Geometry: final body of the model. Coordinates: model frame, mm. A direction names the side the tool comes from. Coordinates: 2 decimals unless noted, no trailing zeros. Write each loop counter-clockwise with the first axis right and the second up, starting at its lowest first coordinate (ties: lowest second). Pieces come first, ordered by that corner, then holes. Notation, with made-up numbers: (13, -31) -> (64, -31) arc R16 cw to (64, 0) -> close; hole circle Ø11 at (-24.5, 67.5). An arc over 180 degrees is marked (long way). One line per item, written item: value.
```python
from build123d import *

# Parameters (mm, degrees)
SKETCH1_R           = 12.4
BOSS_EXTRUDE1_DEPTH = 7
SKETCH2_R           = 1
CUT_EXTRUDE1_DEPTH  = 19.881737208
WRAP1_START         = -0.5
WRAP1_DEPTH         = 0.5
SKETCH4_R           = 0.5
CUT_EXTRUDE2_DEPTH  = 7


# Read off the part's stored shape, not the designer's step: Wrap1
with BuildPart() as part:
    # Sketch1 → Boss-Extrude1 (new body)
    with BuildSketch(Plane(origin=(0, 0, 0), x_dir=(1, 0, 0), z_dir=(0, 1, 0))):
        with Locations(Location((0, 0, 0), (0, 0, 270))):
            Circle(SKETCH1_R)
    extrude(amount=BOSS_EXTRUDE1_DEPTH)

    # Sketch2 → Cut-Extrude1 (cut, through all)
    with BuildSketch(Plane(origin=(0, 0, 0), x_dir=(-1, 0, 0), z_dir=(0, -1, 0))):
        with Locations(Location((0, 9.7, 0), (0, 0, 90))):
            Circle(SKETCH2_R)
        with Locations(Location((0, -9.7, 0), (0, 0, 90))):
            Circle(SKETCH2_R)
    extrude(amount=-CUT_EXTRUDE1_DEPTH, mode=Mode.SUBTRACT)

    # Wrap1 outline → Wrap1 (cut)
    # profile 1 of 6: a face of its own
    with BuildSketch(Plane.XZ.offset(WRAP1_START)):
        with BuildLine():
            Line((-2.031477868, -3.153846154), (-2.210263925, -3.153846154))
            add(Edge.make_bspline(
                [(-2.210263925, -3.153846154), (-2.304050451, -3.153758336), (-2.51704944, -3.153558894), (-2.728459302, -3.180072549), (-2.846782355, -3.194911859)],
                knots=[0, 0, 0, 0, 0.440314414, 1, 1, 1, 1], degree=3))
            add(Edge.make_bspline(
                [(-2.846782355, -3.194911859), (-2.973262529, -3.243260598), (-3.258825144, -3.352420729), (-3.314541645, -3.658766612), (-3.345580432, -3.829427083)],
                knots=[0, 0, 0, 0, 0.442915733, 1, 1, 1, 1], degree=3))
            add(Edge.make_bspline(
                [(-3.345580432, -3.829427083), (-3.329443977, -3.960601874), (-3.292993392, -4.25691217), (-3.019329137, -4.388888631), (-2.866814406, -4.462439904)],
                knots=[0, 0, 0, 0, 0.442694001, 1, 1, 1, 1], degree=3))
            add(Edge.make_bspline(
                [(-2.866814406, -4.462439904), (-2.783809352, -4.4741997), (-2.595026902, -4.500945579), (-2.404280932, -4.500339561), (-2.297403348, -4.5)],
                knots=[0, 0, 0, 0, 0.439686282, 1, 1, 1, 1], degree=3))
            Line((-2.297403348, -4.5), (-1.807118893, -4.5))
            Line((-1.807118893, -4.5), (-1.807118893, -2))
            Line((-1.807118893, -2), (-2.031477868, -2))
            Line((-2.031477868, -2), (-2.031477868, -3.153846154))
        make_face()
        with BuildLine():
            Line((-2.031477868, -4.243589744), (-2.488709438, -4.243589744))
            add(Edge.make_bspline(
                [(-2.488709438, -4.243589744), (-2.636778663, -4.245832648), (-2.858668728, -4.249193765), (-3.087398478, -4.043591474), (-3.109947004, -3.900148285), (-3.121221457, -3.828425481)],
                knots=[0, 0, 0, 0, 0.500718692, 0.750355136, 1, 1, 1, 1], degree=3))
            add(Edge.make_bspline(
                [(-3.121221457, -3.828425481), (-3.110084042, -3.754426269), (-3.087818883, -3.606492103), (-2.846982746, -3.401705038), (-2.620432253, -3.403529508), (-2.469178188, -3.404747596)],
                knots=[0, 0, 0, 0, 0.249615048, 0.499013341, 1, 1, 1, 1], degree=3))
            Line((-2.469178188, -3.404747596), (-2.031477868, -3.41025641))
            Line((-2.031477868, -3.41025641), (-2.031477868, -4.243589744))
        make_face(mode=Mode.SUBTRACT)
    # profile 2 of 6: a face of its own
    with BuildSketch(Plane.XZ.offset(WRAP1_START)):
        with BuildLine():
            add(Edge.make_bspline(
                [(-1.29429838, -3.251001603), (-1.233767931, -3.555711086), (-1.13419239, -4.056973037), (-0.546785242, -4.501043755), (-0.158404316, -4.54307981), (0.035829825, -4.564102564)],
                knots=[0, 0, 0, 0, 0.436607301, 0.718240291, 1, 1, 1, 1], degree=3))
            add(Edge.make_bspline(
                [(0.035829825, -4.564102564), (0.337186775, -4.501451173), (0.832784511, -4.398417587), (1.263646175, -3.813137767), (1.310482432, -3.430401214), (1.333906748, -3.238982372)],
                knots=[0, 0, 0, 0, 0.436786424, 0.718318801, 1, 1, 1, 1], degree=3))
            add(Edge.make_bspline(
                [(1.333906748, -3.238982372), (1.271523902, -2.938761966), (1.168876948, -2.444768626), (0.592223534, -2.001267596), (0.207932181, -1.957686637), (0.015797773, -1.935897436)],
                knots=[0, 0, 0, 0, 0.436529586, 0.718281316, 1, 1, 1, 1], degree=3))
            add(Edge.make_bspline(
                [(0.015797773, -1.935897436), (-0.285288336, -1.99709136), (-0.780661114, -2.09777287), (-1.227049335, -2.673889596), (-1.271884529, -3.058652359), (-1.29429838, -3.251001603)],
                knots=[0, 0, 0, 0, 0.436613243, 0.71835368, 1, 1, 1, 1], degree=3))
        make_face()
        with BuildLine():
            add(Edge.make_bspline(
                [(0.024812197, -4.307692308), (-0.222096477, -4.260150518), (-0.627501361, -4.182090587), (-1.011681906, -3.724534497), (-1.050518548, -3.409193504), (-1.069939406, -3.251502404)],
                knots=[0, 0, 0, 0, 0.437825955, 0.718876246, 1, 1, 1, 1], degree=3))
            add(Edge.make_bspline(
                [(-1.069939406, -3.251502404), (-1.019780636, -3.002340488), (-0.937269286, -2.592468281), (-0.447437557, -2.247759346), (-0.132657177, -2.210797775), (0.024812197, -2.192307692)],
                knots=[0, 0, 0, 0, 0.43655613, 0.718136331, 1, 1, 1, 1], degree=3))
            add(Edge.make_bspline(
                [(0.024812197, -2.192307692), (0.269360953, -2.239222325), (0.671380896, -2.316346488), (1.051425571, -2.770762078), (1.090179676, -3.083624875), (1.109547773, -3.239983974)],
                knots=[0, 0, 0, 0, 0.437205081, 0.718732595, 1, 1, 1, 1], degree=3))
            add(Edge.make_bspline(
                [(1.109547773, -3.239983974), (1.059317235, -3.487706151), (0.97667219, -3.89528709), (0.494781539, -4.245984232), (0.181454127, -4.287124855), (0.024812197, -4.307692308)],
                knots=[0, 0, 0, 0, 0.436595419, 0.718336864, 1, 1, 1, 1], degree=3))
        make_face(mode=Mode.SUBTRACT)
    # profile 3 of 6: a face of its own
    with BuildSketch(Plane.XZ.offset(WRAP1_START)):
        Polygon((1.654419568, -4.5), (2.968522132, -4.5), (2.968522132, -4.243589744), (2.423650338, -4.243589744), (2.423650338, -2), (2.199291363, -2), (2.199291363, -4.243589744), (1.654419568, -4.243589744), align=None)
    # profile 4 of 6: a face of its own
    with BuildSketch(Plane.XZ.offset(WRAP1_START)):
        Polygon((0, -8.309401077), (2, -4.845299462), (-2, -4.845299462), align=None)
    # profile 5 of 6: a face of its own
    with BuildSketch(Plane.XZ.offset(WRAP1_START)):
        Polygon((-2, 4.845299462), (2, 4.845299462), (0, 8.309401077), align=None)
    # profile 6 of 6: a face of its own
    with BuildSketch(Plane.XZ.offset(WRAP1_START)):
        Polygon((0, -11.777350269), (0.5, -10.911324865), (-0.5, -10.911324865), align=None)
    extrude(amount=WRAP1_DEPTH, mode=Mode.SUBTRACT)

    # Sketch4 → Cut-Extrude2 (cut)
    with BuildSketch(Plane(origin=(0, 0, 0), x_dir=(-1, 0, 0), z_dir=(0, -1, 0))):
        with Locations((0, 12.4)):
            Circle(SKETCH4_R)
    extrude(amount=-CUT_EXTRUDE2_DEPTH, mode=Mode.SUBTRACT)


solid = part.part
```
(1) Section C-C (x = 3.5). Return the cut outline in (y, z).
Responses:
outline: (0, -11.9) -> (7, -11.9) -> (7, 11.9) -> (0, 11.9) -> close
(2) Pull-direction query (X, two-part tool) for faces 1 (the flat face through (-2.6, 0, -3.8)), 2 (the flat face through (0.986, 0.254, -6.602)); classes: released by +X, released by -X, zero draft, split by the parting line, or undercut.
Responses:
face 1: zero draft
face 2: undercut
(3) Section B-B (y = 5.25). Return the cut outline in (x, z), then the cut area to 3 significant figures.
Responses:
outline: (-0.5, -12.39) arc R0.5 cw to (0.5, -12.39) arc R12.4 ccw (long way) to start; hole circle Ø2 at (0, -9.7); hole circle Ø2 at (0, 9.7)
area: 476 mm2
(4) Section D-D (z = -6.75). Return the cut outline in (x, y).
Responses:
outline: (-10.4, 0) -> (-0.9, 0) -> (-0.9, 0.5) -> (0.9, 0.5) -> (0.9, 0) -> (10.4, 0) -> (10.4, 7) -> (-10.4, 7) -> close
(5) Section A-A (z = 9.25). Return the cut outline in (x, y), then the cut area to 3 significant figures.
Responses:
outline: (-8.26, 0) -> (-0.89, 0) -> (-0.89, 7) -> (-8.26, 7) -> close; (0.89, 0) -> (8.26, 0) -> (8.26, 7) -> (0.89, 7) -> close
area: 103 mm2
(6) First-contact query: pin 1 (3 mm diameter, centred on y = 5, z = -6.5, fed in from -X); pin 2 (0.6 mm diameter, centred on x = -0.5, y = 0, fed in from +Z). Flat tips, straight axial feed; report the tip coordinate or a pass-through.
Responses:
pin 1: stops at x = -11.35
pin 2: stops at z = 12.4
(7) Line query: line 1 (X direction, y = 1.75, z = -9.7); line 2 (X direction, y = 3.75, z = -10.25); line 3 (X direction, y = 5, z = -8). Output: solid intervals per line, ascending. Write a range as [from, to].
Responses:
line 1: x = [-7.72, -1], [1, 7.72]
line 2: x = [-6.98, -0.84], [0.84, 6.98]
line 3: x = [-9.47, 9.47]
(8) Reachability of faces 3 (the cylindrical face through (0, 3.5, -11.9)), 4 (the flat face through (0, 0.5, 6)) from +Z, -Z, +X, -X, +Y, -Y: full face, straight path, thin tool, end or side. Return the list, or none.
Responses:
face 3: -Z, +Y, -Y
face 4: -Y
